```python
from build123d import *

# Parameters (mm, degrees)
SKETCH1_R           = 17.95
BOSS_EXTRUDE1_DEPTH = 50.5
SKETCH2_R           = 3
BOSS_EXTRUDE2_DEPTH = 37
SKETCH3_W           = 71.5
SKETCH3_H           = 22
SKETCH3_R           = 4.5
BOSS_EXTRUDE3_DEPTH = 7
SKETCH4_W           = 11
SKETCH4_H           = 22
BOSS_EXTRUDE4_DEPTH = 4
SKETCH5_R           = 2
CUT_EXTRUDE1_DEPTH  = 11
SKETCH6_W           = 1.486858086
SKETCH6_H           = 8.145396468
SKETCH6_W_2         = 1.874734108
BOSS_EXTRUDE6_DEPTH = 7


with BuildPart() as part:
    # Sketch1 → Boss-Extrude1 (new body)
    with BuildSketch(Plane.XY):
        Circle(SKETCH1_R)
    extrude(amount=BOSS_EXTRUDE1_DEPTH)

    # Sketch2 → Boss-Extrude2 (add)
    with BuildSketch(Plane.XY.offset(50.5)):
        Circle(SKETCH2_R)
    extrude(amount=BOSS_EXTRUDE2_DEPTH)

    # Sketch3 → Boss-Extrude3 (add)
    with BuildSketch(Plane.XY.offset(50.5)):
        Rectangle(SKETCH3_W, SKETCH3_H)
        Circle(SKETCH3_R, mode=Mode.SUBTRACT)
    extrude(amount=BOSS_EXTRUDE3_DEPTH)

    # Sketch4 → Boss-Extrude4 (add)
    with BuildSketch(Plane.XY.offset(57.5)):
        with Locations((-30.25, 0)):
            Rectangle(SKETCH4_W, SKETCH4_H)
        with Locations((30.25, 0)):
            Rectangle(SKETCH4_W, SKETCH4_H)
    extrude(amount=BOSS_EXTRUDE4_DEPTH)

    # Sketch5 → Cut-Extrude1 (cut)
    with BuildSketch(Plane.XY.offset(61.5)):
        with Locations((-30.25, 6)):
            Circle(SKETCH5_R)
        with Locations((-30.25, -6)):
            Circle(SKETCH5_R)
        with Locations((30.25, -6)):
            Circle(SKETCH5_R)
        with Locations((30.25, 6)):
            Circle(SKETCH5_R)
    extrude(amount=-CUT_EXTRUDE1_DEPTH, mode=Mode.SUBTRACT)

    # Sketch6 → Boss-Extrude6 (add)
    with BuildSketch(Plane(origin=(0, 0, 0), x_dir=(-1, 0, 0), z_dir=(0, 0, -1))):
        with Locations((-13.9312138, 0.937367054)):
            Rectangle(SKETCH6_W, SKETCH6_H)
        with Locations((13.090815752, 0.937367054)):
            Rectangle(SKETCH6_W_2, SKETCH6_H)
    extrude(amount=BOSS_EXTRUDE6_DEPTH)


solid = part.part
```
Read the model definition and answer for the solid it produces. Units are mm, in the model's axes. A direction names the side the tool comes from. Coordinates: 2 decimals unless noted, no trailing zeros. Loops run counter-clockwise (first coordinate to the right, second up) from the corner with the lowest first, then second, coordinate; pieces in that order, holes last. Notation, with made-up numbers: (59, 37.25) - (89, 37.25) arc R19 cw to (89, 48.25) - close; hole circle Ø1 at (44.5, -9). An arc over 180 degrees is marked (long way). Answer in a Markdown table with one row per item.
1. Straight lines are drawn through the part: line 1 (Y direction, x = 30.25, z = 59.25); line 2 (Y direction, x = 0, z = 52.25); line 3 (Z direction, x = 8.5, y = 11.5). For each, find the intervals that lie inside material, in ascending order.
Conclusion:
| item | result |
|---|---|
| line 1 | y = -11 to -8, -4 to 4, 8 to 11 |
| line 2 | y = -11 to -4.5, -3 to 3, 4.5 to 11 |
| line 3 | z = 0 to 50.5 |
2. Find section D-D, the plane x = 0. Write down the section's boundary in (y, z), then the cut area to 3 significant figures.
Conclusion:
| item | result |
|---|---|
| outline | (-17.95, 0) - (17.95, 0) - (17.95, 50.5) - (11, 50.5) - (11, 57.5) - (4.5, 57.5) - (4.5, 50.5) - (3, 50.5) - (3, 87.5) - (-3, 87.5) - (-3, 50.5) - (-4.5, 50.5) - (-4.5, 57.5) - (-11, 57.5) - (-11, 50.5) - (-17.95, 50.5) - close |
| area | 2,130 mm² |
3. Find section A-A, the plane z = 53. Write down the section's boundary in (x, y), then the cut area to 3 significant figures.
Conclusion:
| item | result |
|---|---|
| outline | (-35.75, -11) - (35.75, -11) - (35.75, 11) - (-35.75, 11) - close; circle Ø6 at (0, 0); hole circle Ø4 at (-30.25, -6); hole circle Ø4 at (-30.25, 6); hole circle Ø9 at (0, 0); hole circle Ø4 at (30.25, -6); hole circle Ø4 at (30.25, 6) |
| area | 1,490 mm² |
4. Determine the mould class of faces 1 (the face through (-13, -3.135, -3)), 2 (the face through (35.75, 0, 56)), 3 (the face through (32.158, 6.601, 56.077)) for opening direction Y: +Y half, -Y half, draft (parallel to the pull), parting line (faces both ways), or undercut.
Conclusion:
| item | result |
|---|---|
| face 1 | -Y half |
| face 2 | draft |
| face 3 | undercut |
5. Which of the six approach directions +Z, -Z, +X, -X, +Y, -Y give full straight-line access (tool end or side, diameter ignored) to faces 4 (the face through (0, -14, 50.5)), 5 (the face through (0, 14, 50.5)), 6 (the face through (-30, 0, 61.5)), 7 (the face through (17.12, 5.39, 24.9))?
Conclusion:
| item | result |
|---|---|
| face 4 | +Z, +X, -X, -Y |
| face 5 | +Z, +X, -X, +Y |
| face 6 | +Z, -X, +Y, -Y |
| face 7 | -Z |
6. Find section C-C, the plane y = -6. Write down the section's boundary in (x, z).
Conclusion:
| item | result |
|---|---|
| outline | (-35.75, 50.5) - (-32.25, 50.5) - (-32.25, 61.5) - (-35.75, 61.5) - close; (-28.25, 50.5) - (-16.92, 50.5) - (-16.92, 0) - (16.92, 0) - (16.92, 50.5) - (28.25, 50.5) - (28.25, 61.5) - (24.75, 61.5) - (24.75, 57.5) - (-24.75, 57.5) - (-24.75, 61.5) - (-28.25, 61.5) - close; (32.25, 50.5) - (35.75, 50.5) - (35.75, 61.5) - (32.25, 61.5) - close |
7. Given pin 1 (4.5 mm diameter, centred on x = 30.25, y = 6, fed in from +Z); pin 2 (0.6 mm diameter, centred on x = -13.5, z = -5, fed in from -Y); pin 3 (10 mm diameter, centred on x = 11.5, y = -1.5, fed in from +Z); pin 4 (4 mm diameter, centred on x = 21.5, z = 17, fed in from -Y), each flat-ended and moving along its own axis, determine where each tip first touches the part or whether it passes through.
Conclusion:
| item | result |
|---|---|
| pin 1 | stops at z = 61.5 |
| pin 2 | stops at y = -3.14 |
| pin 3 | stops at z = 57.5 |
| pin 4 | passes through |
8. Find section B-B, the plane x = 30.25. Write down the section's boundary in (y, z), then the cut area to 3 significant figures.
Conclusion:
| item | result |
|---|---|
| outline | (-11, 50.5) - (-8, 50.5) - (-8, 61.5) - (-11, 61.5) - close; (-4, 50.5) - (4, 50.5) - (4, 61.5) - (-4, 61.5) - close; (8, 50.5) - (11, 50.5) - (11, 61.5) - (8, 61.5) - close |
| area | 154 mm² |
